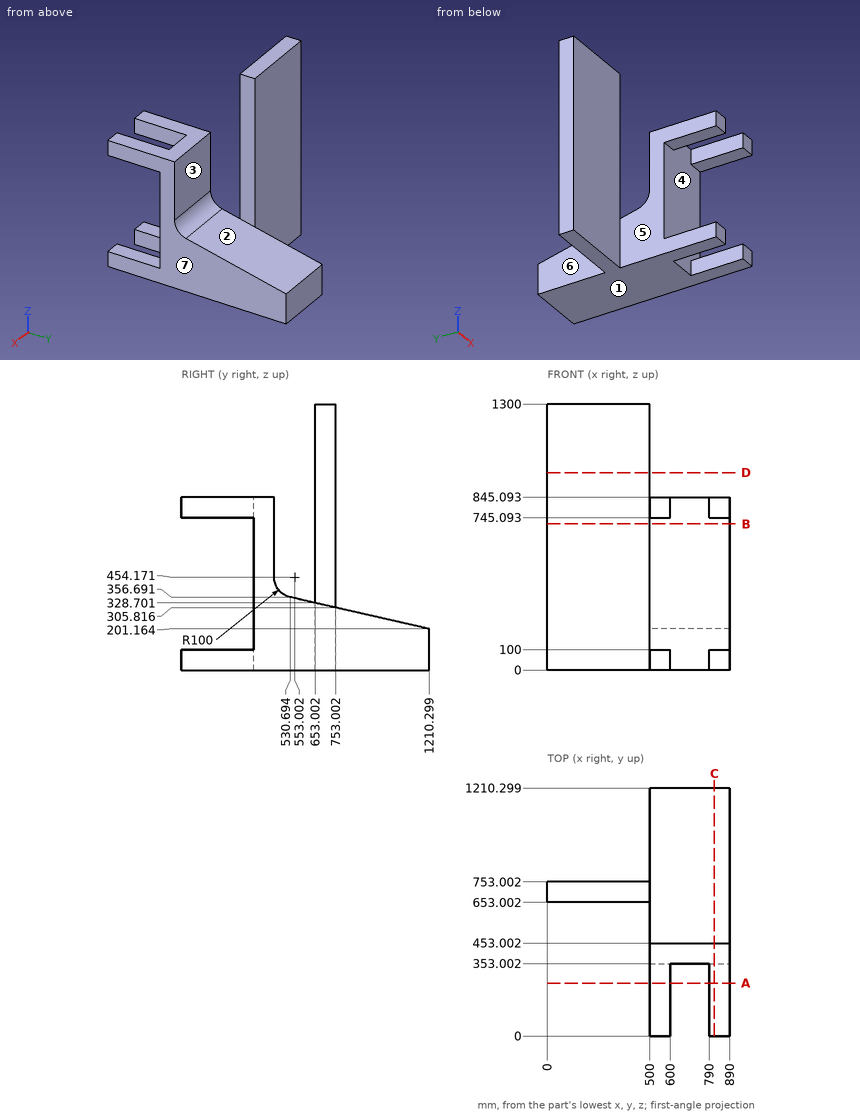
For this review, use the dimensioned drawing (mm, ordinates from the lowest corner) and the shaded views. A direction names the side the tool comes from. Give positions to 0.01 mm unless a question says otherwise; leave off trailing zeros. Order: outer loops, then holes, each group sorted by start corner. A loop starts at its lowest first (then second) coordinate and runs counter-clockwise, first axis right, second up. Notation, with made-up numbers: (76, -1.5) -> (124, -1.5) arc R17 cw to (124, 18.5) -> close; hole circle Ø1 at (-26.5, 25.5). An arc over 180 degrees is marked (long way). Write item = value, one per line. Start each with the question number.
(1) For pin 1 Ø2 at (x, z) = (308.5, 412) entering from -Y; pin 2 Ø12 at (x, z) = (171.5, 402) entering from +Y, all flat-tipped, find the tip position at first contact; note any pin that passes through.
(2) Take a section at A-A (y = 258). Write out the cut boundary in (x, z), plus the area to 3 significant figures.
(3) Take a section at B-B (z = 714.5). Write out the cut boundary in (x, y).
(4) Tool access review of the marked faces 5, 6 and 7: name each direction out of +Z, -Z, +X, -X, +Y, -Y from which nothing blocks a thin tool from reaching the whole face with its end or side.
(5) Take a section at D-D (z = 965). Write out the cut boundary in (x, y), plus the area to 3 significant figures.
(6) Take a section at C-C (x = 816). Write out the cut boundary in (y, z) (1 decimal), plus the area to 3 significant figures.
(7) Draft analysis for pull direction Z (two halves, no side actions). For the marked faces 1, 2, 3 and 4, state which applies: +Z half, -Z half, draft (parallel to the pull), parting line (faces both ways), or undercut.
(8) For L1, parallel to Y at x = 563, z = 476.5; L2, parallel to X at y = 712, z = 830; L3, parallel to X at y = 205, z = 785.5, list the stretches that pass through material, from the lowest coordinate up. Write a range as from..to.
Returned:
q1.pin_1 = 653
q1.pin_2 = 753
q2.outline = (500, 0) -> (600, 0) -> (600, 100) -> (500, 100) -> close; (500, 745.09) -> (600, 745.09) -> (600, 845.09) -> (500, 845.09) -> close; (790, 0) -> (890, 0) -> (890, 100) -> (790, 100) -> close; (790, 745.09) -> (890, 745.09) -> (890, 845.09) -> (790, 845.09) -> close
q2.area = 40,000 mm²
q3.outline = (0, 653) -> (500, 653) -> (500, 753) -> (0, 753) -> close; (500, 353) -> (890, 353) -> (890, 453) -> (500, 453) -> close
q4.face_5 = +Z, -Z, -X, -Y
q4.face_6 = +Z, -Z, -X, +Y
q4.face_7 = +Z, -Z, +X, +Y, -Y
q5.outline = (0, 653) -> (500, 653) -> (500, 753) -> (0, 753) -> close
q5.area = 50,000 mm²
q6.outline = (0, 0) -> (1210.3, 0) -> (1210.3, 201.2) -> (530.7, 356.7) arc R100 cw to (453, 454.2) -> (453, 845.1) -> (0, 845.1) -> (0, 745.1) -> (353, 745.1) -> (353, 100) -> (0, 100) -> close
q6.area = 374,000 mm²
q7.face_1 = -Z half
q7.face_2 = +Z half
q7.face_3 = draft
q7.face_4 = undercut
q8.L1 = 353..453
q8.L2 = 0..500
q8.L3 = 500..600, 790..890
